Study the drawing (mm; zero at the part's minimum x, y, z) and answer. A direction names the side the tool comes from. Coordinates: 2 decimals unless noted, no trailing zeros. Order: outer loops, then holes, each group sorted by start corner. A loop starts at its lowest first (then second) coordinate and runs counter-clockwise, first axis right, second up.
1. Flat-ended cylindrical pins translate along their axes: pin 1 Ø1.9 at (x, z) = (2.5, 3) entering from +Y; pin 2 Ø5 at (x, z) = (11.5, 10.5) entering from -Y; pin 3 Ø4 at (y, z) = (48, 6) entering from +X (1 decimal); pin 4 Ø1.9 at (y, z) = (2, 5.5) entering from -X. Find the tip coordinate at first contact, or state that the pin passes through.
2. The part is cut by section A-A, the plane y = 25.05. Give the vertices of the cut face in (x, z), then the cut area to 3 significant figures.
3. The part is cut by section D-D, the plane y = 40.05. Give the vertices of the cut face in (x, z).
4. Determine the mould class of the marked faces 1, 2 and 3 for opening direction Y: +Y half, -Y half, draft (parallel to the pull), parting line (faces both ways), or undercut.
5. A tool of negligible diameter and unlimited length cuts with its end or side. For the marked faces 4, 5, 6 and 7, from which of +Z, -Z, +X, -X, +Y, -Y can it reach the whole face along a straight path? Write none if from no direction.
6. Find the intervals of material crossed by probe 1 along Y at (x, z) = (25.05, 6); probe 2 along Z at (x, y) = (9, 17.5); probe 3 along Y at (x, z) = (10, 10.25), in increasing order.
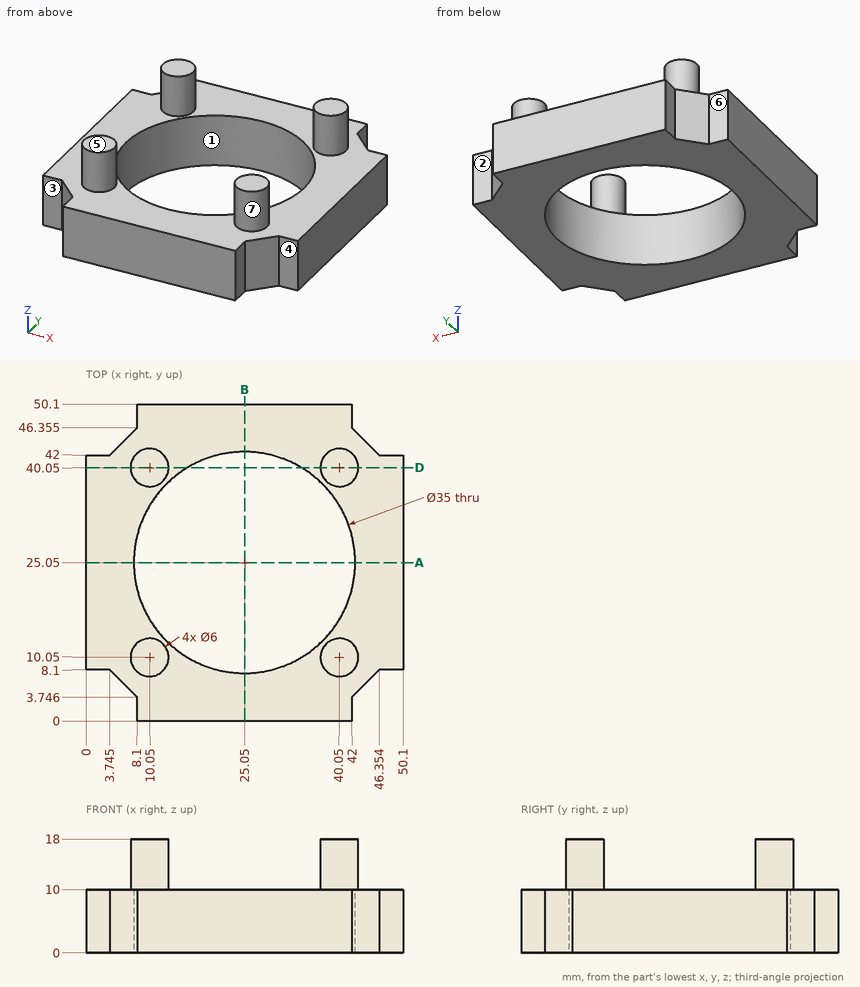
Geometry says:
1. pin 1: stops at y = 42
1. pin 2: stops at y = 0
1. pin 3: stops at x = 42.4
1. pin 4: stops at x = 8.1
2. outline: (0, 0) - (7.55, 0) - (7.55, 10) - (0, 10) - close; (42.55, 0) - (50.1, 0) - (50.1, 10) - (42.55, 10) - close
2. area: 151 mm2
3. outline: (0, 0) - (16.04, 0) - (16.04, 10) - (13.05, 10) - (13.05, 18) - (7.05, 18) - (7.05, 10) - (0, 10) - close; (34.06, 0) - (50.1, 0) - (50.1, 10) - (43.05, 10) - (43.05, 18) - (37.05, 18) - (37.05, 10) - (34.06, 10) - close
4. face 1: undercut
4. face 2: +Y half
4. face 3: -Y half
5. face 4: +Z, -Z, +X, -Y
5. face 5: +Z, +X, -X, +Y, -Y
5. face 6: +Z, -Z, -X, +Y
5. face 7: +Z
6. probe 1: y = 0 to 7.55, 42.55 to 50.1
6. probe 2: z = 0 to 10
6. probe 3: y = 7.05 to 13.05, 37.05 to 43.05
